Could you check a few things on this model? Use its own coordinates, in mm. Face numbers are marked on the shaded views. Give positions to 0.01 mm unless a question says otherwise; leave off trailing zeros. Loops run counter-clockwise (first coordinate to the right, second up) from the corner with the lowest first, then second, coordinate; pieces in that order, holes last. Notation, with made-up numbers: (59.5, 65) - (78.5, 65) arc R25 cw to (78.5, 104) - close; hole circle Ø11 at (83.5, -39). An arc over 180 degrees is marked (long way). Answer in a Markdown table with one row per item. Add a question column.
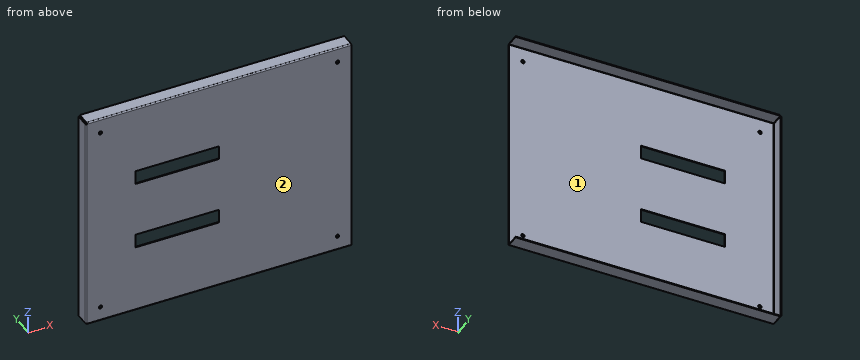
```python
from build123d import *

# Parameters (mm, degrees)
SKETCH3_W          = 482.5780122
SKETCH3_H          = 398.4879
BASE_FLANGE1_DEPTH = 1.5875
EDGE_FLANGE1_DEPTH = 482.5780122
EDGE_FLANGE2_DEPTH = 482.5780122
EDGE_FLANGE4_DEPTH = 398.4879
SKETCH20_W         = 152.4
SKETCH20_H         = 25.4
CUT_EXTRUDE1_DEPTH = 1.5875
SKETCH21_R         = 3.175
CUT_EXTRUDE2_DEPTH = 1.5875


# Sheet-metal steps are written as plain solids
with BuildPart() as part:
    # Sketch3 → Base-Flange1 (new body)
    with BuildSketch(Plane(origin=(0, 0, 0), x_dir=(1, 0, 0), z_dir=(0, 1, 0))):
        with Locations((241.2890061, 199.24395)):
            Rectangle(SKETCH3_W, SKETCH3_H)
    extrude(amount=-BASE_FLANGE1_DEPTH)

    # Edge-Flange1 section (across the edge) → Edge-Flange1 (add)
    with BuildSketch(Plane(origin=(0, 0, 0.7366), x_dir=(0, 0, -1), z_dir=(1, 0, 0))):
        with BuildLine():
            Line((-1.5875, 0.7366), (-1.5875, 23.8125))
            Line((-1.5875, 23.8125), (0, 23.8125))
            Line((0, 23.8125), (0, 0.7366))
            ThreePointArc((0, 0.7366), (0.215745145, 0.215745145), (0.7366, 0))
            Line((0.7366, 0), (0.7366, -1.5875))
            ThreePointArc((0.7366, -1.5875), (-0.90678687, -0.90678687), (-1.5875, 0.7366))
        make_face()
    extrude(amount=EDGE_FLANGE1_DEPTH)

    # Edge-Flange2 section (across the edge) → Edge-Flange2 (add)
    with BuildSketch(Plane(origin=(482.5780122, 0, -399.2245), x_dir=(0, 0, 1), z_dir=(-1, 0, 0))):
        with BuildLine():
            Line((-1.5875, 0.7366), (-1.5875, 23.8125))
            Line((-1.5875, 23.8125), (0, 23.8125))
            Line((0, 23.8125), (0, 0.7366))
            ThreePointArc((0, 0.7366), (0.215745145, 0.215745145), (0.7366, 0))
            Line((0.7366, 0), (0.7366, -1.5875))
            ThreePointArc((0.7366, -1.5875), (-0.90678687, -0.90678687), (-1.5875, 0.7366))
        make_face()
    extrude(amount=EDGE_FLANGE2_DEPTH)

    # Edge-Flange4 section (across the edge) → Edge-Flange4 (add)
    with BuildSketch(Plane(origin=(-0.7366, 0, -398.4879), x_dir=(1, 0, 0), z_dir=(0, 0, 1))):
        with BuildLine():
            Line((-1.5875, 0.7366), (-1.5875, 23.8125))
            Line((-1.5875, 23.8125), (0, 23.8125))
            Line((0, 23.8125), (0, 0.7366))
            ThreePointArc((0, 0.7366), (0.215745145, 0.215745145), (0.7366, 0))
            Line((0.7366, 0), (0.7366, -1.5875))
            ThreePointArc((0.7366, -1.5875), (-0.90678687, -0.90678687), (-1.5875, 0.7366))
        make_face()
    extrude(amount=EDGE_FLANGE4_DEPTH)

    # Sketch20 → Cut-Extrude1 (cut)
    with BuildSketch(Plane(origin=(0, 0, 0), x_dir=(1, 0, 0), z_dir=(0, 1, 0))):
        with Locations((165.0890061, 135.74395)):
            Rectangle(SKETCH20_W, SKETCH20_H)
        with Locations((165.0890061, 262.74395)):
            Rectangle(SKETCH20_W, SKETCH20_H)
    extrude(amount=-CUT_EXTRUDE1_DEPTH, mode=Mode.SUBTRACT)

    # Sketch21 → Cut-Extrude2 (cut)
    with BuildSketch(Plane(origin=(0, 0, 0), x_dir=(1, 0, 0), z_dir=(0, 1, 0))):
        with Locations(Location((24.6634, 373.8245, 0), (0, 0, 270))):
            Circle(SKETCH21_R)
        with Locations(Location((457.1780122, 373.8245, 0), (0, 0, 270))):
            Circle(SKETCH21_R)
        with Locations(Location((457.1780122, 25.4, 0), (0, 0, 270))):
            Circle(SKETCH21_R)
        with Locations(Location((24.6634, 25.4, 0), (0, 0, 270))):
            Circle(SKETCH21_R)
    extrude(amount=-CUT_EXTRUDE2_DEPTH, mode=Mode.SUBTRACT)


solid = part.part
```
(1) We'd pull the mould along Z, two halves only. Please class the marked faces 1 and 2: pulls with the +Z half, pulls with the -Z half, needs draft (parallel to the pull), parting line crosses it, or undercut.
(2) Please list where these lines run through material, in increasing order: line 1 (Z direction, x = 49.5, y = 22.5); line 2 (X direction, y = -1.2, z = -25.4); line 3 (X direction, y = 12.75, z = -302).
(3) I want a section at B-B on x = 225. Please give me the cut outline in (y, z).
(4) For pin 1 Ø1.3 at (x, y) = (136.5, -1) entering from +Z; pin 2 Ø0.5 at (x, y) = (185, -1) entering from -Z; pin 3 Ø1 at (x, z) = (253.5, -168) entering from +Y; pin 4 Ø5.5 at (x, z) = (457.18, -25.4) entering from -Y, each with a flat end and sliding along its axis, tell me the tip position at first contact or that it passes through.
(5) I want a section at D-D on z = -56.5. Please give me the cut outline in (x, y).
(6) I want a section at C-C on x = 432. Please give me the cut outline in (y, z).
(7) I want a section at A-A on y = 5. Please give me the cut outline in (x, z), then the cut area to 3 significant figures.
Reported:
| question | item | result |
|---|---|---|
| 1 | face 1 | undercut |
| 1 | face 2 | needs draft |
| 2 | line 1 | -400.81 to -399.22, 0.74 to 2.32 |
| 2 | line 2 | -1.28 to 21.49, 27.84 to 454, 460.35 to 482.58 |
| 2 | line 3 | -2.32 to -0.74 |
| 3 | outline | (-1.59, -398.49) arc R2.32 ccw to (0.74, -400.81) - (23.81, -400.81) - (23.81, -399.22) - (0.74, -399.22) arc R0.74 cw to (0, -398.49) - (0, -275.44) - (-1.59, -275.44) - close; (-1.59, -250.04) - (0, -250.04) - (0, -148.44) - (-1.59, -148.44) - close; (-1.59, -123.04) - (0, -123.04) - (0, 0) arc R0.74 cw to (0.74, 0.74) - (23.81, 0.74) - (23.81, 2.32) - (0.74, 2.32) arc R2.32 ccw to (-1.59, 0) - close |
| 4 | pin 1 | z = 2.05 |
| 4 | pin 2 | z = -400.27 |
| 4 | pin 3 | y = 0 |
| 4 | pin 4 | through |
| 5 | outline | (-2.32, 0.74) arc R2.32 ccw to (0, -1.59) - (482.58, -1.59) - (482.58, 0) - (0, 0) arc R0.74 cw to (-0.74, 0.74) - (-0.74, 23.81) - (-2.32, 23.81) - close |
| 6 | outline | (-1.59, -398.49) arc R2.32 ccw to (0.74, -400.81) - (23.81, -400.81) - (23.81, -399.22) - (0.74, -399.22) arc R0.74 cw to (0, -398.49) - (0, 0) arc R0.74 cw to (0.74, 0.74) - (23.81, 0.74) - (23.81, 2.32) - (0.74, 2.32) arc R2.32 ccw to (-1.59, 0) - close |
| 7 | outline | (-2.32, -398.49) - (-0.74, -398.49) - (-0.74, 0) - (-2.32, 0) - close; (0, -400.81) - (482.58, -400.81) - (482.58, -399.22) - (0, -399.22) - close; (0, 0.74) - (482.58, 0.74) - (482.58, 2.32) - (0, 2.32) - close |
| 7 | area | 2,160 mm² |
